Here's how the part is built. I have some questions about the finished solid (model axes, mm). A direction names the side the tool comes from. Give positions to 0.01 mm unless a question says otherwise; leave off trailing zeros. Loops run counter-clockwise (first coordinate to the right, second up) from the corner with the lowest first, then second, coordinate; pieces in that order, holes last. Notation, with made-up numbers: (-30.75, 60.5) - (27.25, 60.5) arc R18 ccw to (27.25, 90.5) - close; hole circle Ø10 at (61.25, -4). An arc over 180 degrees is marked (long way). One line per item, written item: value. Start each with the question number.
```python
from build123d import *

# Parameters (mm, degrees)
F0_W      = 762
F0_H      = 660.4
F1_DEPTH  = 25.4
F2_W      = 508
F2_H      = 279.4
F3_DEPTH  = 228.6
F4_W      = 254
F4_H      = 152.4
F5_DEPTH  = 2.54
F6_W      = 254
F6_H      = 228.6
F7_DEPTH  = 25.4
F8_W      = 76.2
F8_H      = 152.4
F8_H_2    = 177.8
F9_DEPTH  = 2.54
F11_W     = 152.4
F11_H     = 152.4
F12_DEPTH = 2.54
F13_W     = 508
F13_H     = 292.1
F14_DEPTH = 228.6
F16_W     = 254
F16_H     = 25.4
F17_DEPTH = 228.6
F18_DEPTH = 266.7
F20_DEPTH = 266.701
F21_W     = 8.382
F21_H     = 8.382
F22_DEPTH = 228.6


with BuildPart() as f1:
    # F0 (on Top) → F1 (new body)
    with BuildSketch(Plane.XY):
        Rectangle(F0_W, F0_H)
    extrude(amount=-F1_DEPTH)

    # F2 (on face) → F3 (join)
    with BuildSketch(Plane.XY):
        with Locations((127, 190.5)):
            Rectangle(F2_W, F2_H)
    extrude(amount=F3_DEPTH)

    # F4 (on face) → F5 (cut)
    with BuildSketch(Plane.XZ.offset(-50.8)):
        with Locations((127, 152.4)):
            Rectangle(F4_W, F4_H)
    extrude(amount=-F5_DEPTH, mode=Mode.SUBTRACT)

    # F8 (on face) → F9 (cut)
    with BuildSketch(Plane(origin=(-127, 0, 0), x_dir=(0, -1, 0), z_dir=(-1, 0, 0))):
        with Locations((-127, 152.4)):
            Rectangle(F8_W, F8_H)
        with Locations((-254, 88.9)):
            Rectangle(F8_W, F8_H_2)
    extrude(amount=-F9_DEPTH, mode=Mode.SUBTRACT)


with BuildPart() as f7:
    # F6 (on face) → F7 (new body)
    with BuildSketch(Plane(origin=(0, 330.2, 0), x_dir=(-1, 0, 0), z_dir=(0, 1, 0))):
        with Locations((254, 114.3)):
            Rectangle(F6_W, F6_H)
    extrude(amount=-F7_DEPTH)

    # F10: union F1
    add(f1.part)

    # F11 (on face) → F12 (cut)
    with BuildSketch(Plane.XZ.offset(-304.8)):
        with Locations((-254, 152.4)):
            Rectangle(F11_W, F11_H)
    extrude(amount=-F12_DEPTH, mode=Mode.SUBTRACT)

    # F13 (on face) → F14 (join)
    with BuildSketch(Plane.XY.offset(228.6)):
        with Locations((127, 184.15)):
            Rectangle(F13_W, F13_H)
    extrude(amount=F14_DEPTH)

    # F16 (on face) → F17 (join)
    with BuildSketch(Plane.XY.offset(228.6)):
        with Locations((-254, 317.5)):
            Rectangle(F16_W, F16_H)
    extrude(amount=F17_DEPTH)

    # F15 (on face) → F18 (join)
    with BuildSketch(Plane(origin=(-127, 0, 0), x_dir=(0, -1, 0), z_dir=(-1, 0, 0))):
        Polygon((-304.8, 295.9728837013), (-304.8, 228.6), (-38.1, 228.6), align=None)
    extrude(amount=F18_DEPTH)

    # F19 (on face) → F20 (cut, through all)
    with BuildSketch(Plane(origin=(0, 304.8, 0), x_dir=(-1, 0, 0), z_dir=(0, 1, 0))):
        Polygon((127, 295.9728837013), (393.7, 228.6), (393.7, 295.9728837013), align=None)
    extrude(amount=-F20_DEPTH, mode=Mode.SUBTRACT)

    # F21 (on face) → F22 (join)
    with BuildSketch(Plane(origin=(0, 0, 228.6), x_dir=(1, 0, 0), z_dir=(0, 0, -1))):
        with Locations((-351.409, -80.391)):
            Rectangle(F21_W, F21_H)
    extrude(amount=F22_DEPTH)


solid = f7.part
```
(1) Please list where these lines run through material, in increasing order: probe 1 along Y at (x, z) = (293, 43); probe 2 along Y at (x, z) = (102, 228); probe 3 along Z at (x, y) = (-62.5, -220.5). Write a range as from..to.
(2) Will these pins go through, and if not, where does the flat tip stop? pin 1 (1.5 mm diameter, centred on x = -256, z = 352, fed in from -Y); pin 2 (2.5 mm diameter, centred on x = -388, z = 230, fed in from +Y); pin 3 (6.5 mm diameter, centred on y = 78.5, z = 73.5, fed in from -X).
(3) If we section it at B-B on x = -63: List the corners of the cut face in (y, z) for me.
(4) If we section it at D-D on y = -101: List the corners of the cut face in (x, z) for me, plus the area to 3 significant figures.
(5) For faces 4 (the face through (-228.85, 139.95, 254.33)), 5 (the face through (123, 38.1, 341)), 6 (the face through (-124.46, 255, 90)), 7 (the face through (-255, 307.34, 153)), which set-ups out of +Z, -Z, +X, -X, +Y, -Y let a thin tool reach every point of the face, with its end or its side?
(6) If we section it at A-A on z = 90: List the corners of the cut face in (x, y) for me.
(7) If we section it at C-C on z = 355.5: List the corners of the cut face in (x, y) for me, plus the area to 3 significant figures.
(8) If we mould it in two halves opening along Z, with no side actions, what happens to faces 1 (the face through (-256, 304.8, 62)), 2 (the face through (-5, 330.2, 213)), 3 (the face through (-317.7, 232.6, 247.8))? For each: pulls with the +Z half, pulls with the -Z half, needs draft (parallel to the pull), parting line crosses it, or undercut.
Found:
1. probe 1: 50.8..330.2
1. probe 2: 53.34..330.2
1. probe 3: -25.4..0
2. pin 1: y = 304.8
2. pin 2: y = 304.8
2. pin 3: x = -355.6
3. outline: (-330.2, -25.4) - (330.2, -25.4) - (330.2, 457.2) - (38.1, 457.2) - (38.1, 228.6) - (50.8, 228.6) - (50.8, 0) - (-330.2, 0) - close
4. outline: (-381, -25.4) - (381, -25.4) - (381, 0) - (-381, 0) - close
4. area: 19,400 mm^2
5. face 4: +Z, -X, -Y
5. face 5: +Z, +X, -X, -Y
5. face 6: -X
5. face 7: -Y
6. outline: (-381, 304.8) - (-330.2, 304.8) - (-330.2, 307.34) - (-177.8, 307.34) - (-177.8, 304.8) - (-127, 304.8) - (-127, 292.1) - (-124.46, 292.1) - (-124.46, 215.9) - (-127, 215.9) - (-127, 165.1) - (-124.46, 165.1) - (-124.46, 88.9) - (-127, 88.9) - (-127, 50.8) - (0, 50.8) - (0, 53.34) - (254, 53.34) - (254, 50.8) - (381, 50.8) - (381, 330.2) - (-381, 330.2) - close; (-355.6, 76.2) - (-347.22, 76.2) - (-347.22, 84.58) - (-355.6, 84.58) - close
7. outline: (-381, 304.8) - (-127, 304.8) - (-127, 38.1) - (381, 38.1) - (381, 330.2) - (-381, 330.2) - close
7. area: 155,000 mm^2
8. face 1: undercut
8. face 2: needs draft
8. face 3: pulls with the +Z half
